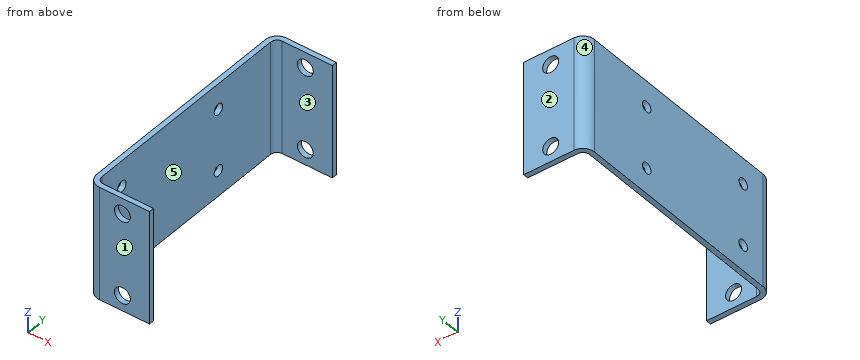
Autodesk Inventor part; units mm, degrees
ref_plane "YZ Plane" through (0, 0, 0) normal (1, 0, 0) x (0, 1, 0)
ref_plane "XZ Plane" through (0, 0, 0) normal (0, 1, 0) x (-1, 0, 0)
ref_plane "XY Plane" through (0, 0, 0) normal (0, 0, 1) x (1, 0, 0)
sketch "Boceto1" plane through (0, 0, 0) normal (1, 0, 0) x (0, 1, 0)
  line L0 (0, 0) -> (46.5, 0)
  line L1 (46.5, 0) -> (46.5, -22)
  line L2 (46.5, -22) -> (0, -22)
  line L3 (0, -22) -> (0, 0)
  dimension "d0" = 46.5
  dimension "d1" = 22
extrude "Placa1" add sketch "Boceto1" along normal blind 1
sketch "Boceto2" plane through (0, 45.5, 0) normal (0, 1, 0) x (-1, 0, 0)
  line L0 (0, -22) -> (0, 0)
  line L1 (0, 0) -> (-12, 0)
  line L2 (-12, 0) -> (-12, -22)
  line L3 (-12, -22) -> (0, -22)
edge flange "Pestaña1" height 12 angle 90 thickness 1 bend radius 1.27 thickness toward (0, 1, 0) relief tear relief width 1 relief depth 0.5 corner gap 1 corner form 0 edges at (1, 46.5, -11) (1, 0, -11) wall of the first edge with corners at (0, 45.5, -22) (0, 45.5, 0) (12, 45.5, 0) (12, 45.5, -22)
bend "Doblez1"
corner "Esquina1"
sketch "Boceto3" plane through (1, 0, 0) normal (1, 0, 0) x (0, 0, -1)
  circle A0 centre (17, 7.25) radius 1.05
  line L0 (0, 0) -> (22, 0)
  line L1 (0, 2.27) -> (0, 44.23)
  line L2 (0, 0) -> (22, 0) construction
  line L3 (11, 0) -> (11, 46.5) construction
  line L4 (22, 46.5) -> (0, 46.5) construction
  circle A1 centre (5, 7.25) radius 1.05
  line L5 (22, 44.23) -> (22, 2.27)
  circle A2 centre (17, 31.25) radius 1.05
  circle A3 centre (5, 31.25) radius 1.05
  dimension "d13" = 2.1
  dimension "d14" = 7.25
  dimension "d16" = 2.1
  dimension "d20" = 24
  dimension "d27" = 12
  dimension "d28" = 6
extrude "Cortar1" cut sketch "Boceto3" against normal blind 1
sketch "Boceto4" plane through (12, 1, 0) normal (0, 1, 0) x (1, 0, 0)
  circle A0 centre (-5.25, 19) radius 1.55
  line L0 (-9.73, 22) -> (0, 22)
  line L1 (0, 0) -> (0, 22) construction
  line L2 (0, 11) -> (-13.2221, 11) construction
  circle A1 centre (-5.25, 3) radius 1.55
  point P0 (-12, 0)
  point P1 (-12, 22)
  dimension "d29" = 3.1
  dimension "d32" = 3
  dimension "d33" = 6.75
extrude "Extrusión1" cut sketch "Boceto4" along normal through all both and the other way through all
equation "\"d25\" = Grosor"
equation "\"d2\" = Grosor"
equation "\"d3\" = Anchura_desahogo_plegado"
equation "\"d4\" = Profundidad_desahogo_plegado"
equation "\"d5\" = Remanente_mínimo"
equation "\"d6\" = Radiodetransición"
equation "\"d10\" = Tamaño_destalonado"
equation "\"d11\" = TamañoSeparación"
equation "\"d12\" = Tamaño_de_radio_de_Jacobi"
equation "\"Radio_pliegue\" = Grosor"
equation "\"Anchura_desahogo_plegado\" = Grosor"
equation "\"Profundidad_desahogo_plegado\" = 0.5 * Grosor"
equation "\"Tamaño_destalonado\" = 4 * Grosor"
equation "\"Remanente_mínimo\" = 2 * Grosor"
equation "\"Radiodetransición\" = Radio_pliegue"
equation "\"Tamaño_de_radio_de_Jacobi\" = Radio_pliegue"
equation "\"TamañoSeparación\" = Grosor"
properties part number "MotorSoport"
Read the model definition and answer for the solid it produces. Units are mm, in the model's axes. Face numbers are marked on the shaded views. A direction names the side the tool comes from. Round coordinates to 2 decimals unless told otherwise and drop trailing zeros. Write each loop counter-clockwise with the first axis right and the second up, starting at its lowest first coordinate (ties: lowest second). Pieces come first, ordered by that corner, then holes. Notation, with made-up numbers: M -20.75,70 L -13.75,70 A23 ccw -13.75,97 Z; hole C 82,-31 d7. An arc over 180 degrees is marked long. Use a Markdown table: item, result.
1) The part is cut by section A-A (z = -5). Write down the section's boundary in (x, y).
Answers follow:
| item | result |
|---|---|
| outline | M 0,2.27 A2.27 ccw 2.27,0 L 12,0 L 12,1 L 2.27,1 A1.27 cw 1,2.27 L 1,6.2 L 0,6.2 Z; M 0,8.3 L 1,8.3 L 1,30.2 L 0,30.2 Z; M 0,32.3 L 1,32.3 L 1,44.23 A1.27 cw 2.27,45.5 L 12,45.5 L 12,46.5 L 2.27,46.5 A2.27 ccw 0,44.23 Z |
2) The part is cut by section C-C (y = 7.25). Write down the section's boundary in (x, z).
Answers follow:
| item | result |
|---|---|
| outline | M 0,-22 L 1,-22 L 1,-18.05 L 0,-18.05 Z; M 0,-15.95 L 1,-15.95 L 1,-6.05 L 0,-6.05 Z; M 0,-3.95 L 1,-3.95 L 1,0 L 0,0 Z |
3) For a pull along Y with two mould halves and no side action, classify the marked faces 1, 2 and 3 as pulls with the +Y half, pulls with the -Y half, needs draft (parallel to the pull), parting line crosses it, or undercut.
Answers follow:
| item | result |
|---|---|
| face 1 | pulls with the -Y half |
| face 2 | pulls with the +Y half |
| face 3 | undercut |
4) A tool of negligible diameter and unlimited length cuts with its end or side. For the marked faces 4 and 5, from which of +Z, -Z, +X, -X, +Y, -Y can it reach the whole face along a straight path? Write none if from no direction.
Answers follow:
| item | result |
|---|---|
| face 4 | +Z, -Z, -X, +Y |
| face 5 | +Z, -Z, +X |
5) Flat-ended cylindrical pins translate along their axes: pin 1 (1 mm diameter, centred on y = 31.5, z = -18.5, fed in from +X); pin 2 (1 mm diameter, centred on x = 1.5, z = -3, fed in from +Y); pin 3 (1.9 mm diameter, centred on y = 31.25, z = -5, fed in from +X). Find the tip coordinate at first contact, or state that the pin passes through.
Answers follow:
| item | result |
|---|---|
| pin 1 | stops at x = 1 |
| pin 2 | stops at y = 46.48 |
| pin 3 | passes through |
6) The part is cut by section B-B (x = 11). Write down the section's boundary in (y, z), plus the area to 3 significant figures.
Answers follow:
| item | result |
|---|---|
| outline | M 0,-22 L 1,-22 L 1,0 L 0,0 Z; M 45.5,-22 L 46.5,-22 L 46.5,0 L 45.5,0 Z |
| area | 44.0 mm2 |
7) The part is cut by section D-D (z = -11.5). Write down the section's boundary in (x, y).
Answers follow:
| item | result |
|---|---|
| outline | M 0,2.27 A2.27 ccw 2.27,0 L 12,0 L 12,1 L 2.27,1 A1.27 cw 1,2.27 L 1,44.23 A1.27 cw 2.27,45.5 L 12,45.5 L 12,46.5 L 2.27,46.5 A2.27 ccw 0,44.23 Z |
8) Straight lines are drawn through the part: line 1 along Z through (x, y) = (6.75, 46.25); line 2 along Y through (x, z) = (2.25, -12); line 3 along Y through (x, z) = (0.45, -5). For each, find the intervals that lie inside material, in ascending order. Write a range as [from, to].
Answers follow:
| item | result |
|---|---|
| line 1 | z = [-22, -20.55], [-17.45, -4.55], [-1.45, 0] |
| line 2 | y = [0, 1], [45.5, 46.5] |
| line 3 | y = [0.91, 6.2], [8.3, 30.2], [32.3, 45.59] |
